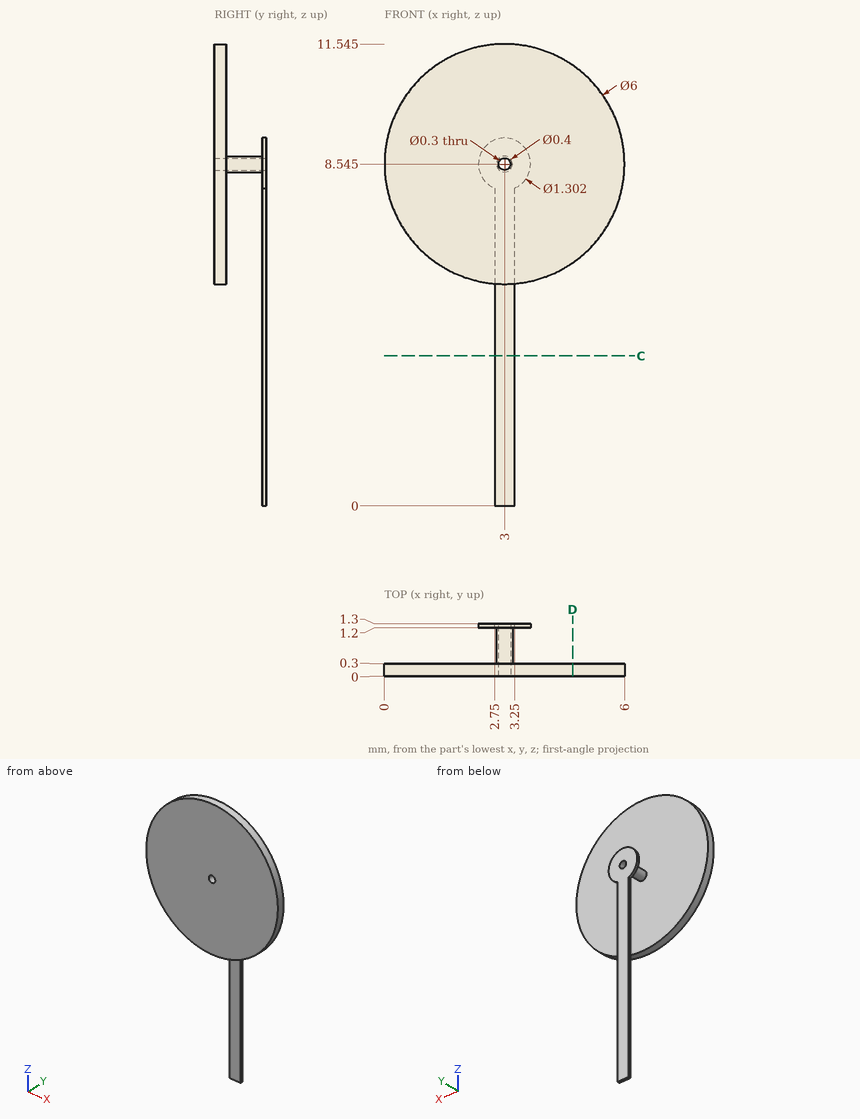
Job drawing, mm, ordinate dimensions from the low corner. One solid piece. Round coordinates to 2 decimals unless told otherwise and drop trailing zeros. Order: outer loops, then holes, each group sorted by start corner. A loop starts at its lowest first (then second) coordinate and runs counter-clockwise, first axis right, second up. Notation, with made-up numbers: (-20.75, 65) -> (-4.75, 65) arc R18 ccw to (-4.75, 94) -> close; hole circle Ø9 at (76, -22). An arc over 180 degrees is marked (long way). Write item = value, one per line.
(1) Cut at D-D (x = 4.7). Write the cut outline in (y, z).
Answers follow:
outline = (0, 6.07) -> (0.3, 6.07) -> (0.3, 11.02) -> (0, 11.02) -> close
(2) Drill centre lines: L1, parallel to Y at x = 1.85, z = 7.25; L2, parallel to Z at x = 2.4, y = 0.1 (1 decimal); L3, parallel to Z at x = 2.1, y = 0.1 (1 decimal). Where is each one in solid material? Low to high.
Answers follow:
L1 = 0 to 0.3
L2 = 5.6 to 11.5
L3 = 5.7 to 11.4
(3) Cut at C-C (z = 3.75). Write the cut outline in (x, y).
Answers follow:
outline = (2.75, 1.2) -> (3.25, 1.2) -> (3.25, 1.3) -> (2.75, 1.3) -> close
